Part model, mm, in its own coordinate system. Coordinates: 2 decimals unless noted, no trailing zeros. Write each loop counter-clockwise with the first axis right and the second up, starting at its lowest first coordinate (ties: lowest second). Pieces come first, ordered by that corner, then holes. Notation, with made-up numbers: M 62,-10 L 70,-10 A21 cw 70,18 Z; hole C 59,-22.5 d8. An arc over 180 degrees is marked long. Use a Markdown table: item, result. Add a question column.
Q1. Pin check, flat tip, straight feed: pin 1 Ø3 at (x, y) = (-114, -21) entering from -Z. Stop position of the tip, or through.
Q2. Slice it at A-A on x = -83. Write the cut outline in (y, z), then the cut area to 3 significant figures.
Q3. Mould opens along X. For faces 1 (the flat face through (-158, -76, 2)), 2 (the flat face through (0, -76, 2)), 3 (the cylindrical face through (-123, -105, 2)) say: released by +X, released by -X, zero draft, split by the parting line, or undercut.
Q4. Slice it at C-C on z = 1. Write the cut outline in (x, y).
Q5. Slice it at B-B on y = -97. Write the cut outline in (x, z), then the cut area to 3 significant figures.
Q6. Wall check: L1, parallel to X at y = -142.5, z = 0.9; L2, parallel to Y at x = -156, z = 2.95; L3, parallel to Y at x = -84, z = 0.7. Give the ranges that are in metal, low to high. Write a range as from..to.
from build123d import *

# Parameters (mm, degrees)
F0_W     = 158
F0_H     = 150
F1_DEPTH = 4
F2_R     = 1.5
F3_DEPTH = 25
F4_R     = 50
F5_DEPTH = 25


with BuildPart() as f1:
    # F0 (on Top) → F1 (new body)
    with BuildSketch(Plane.XY):
        with Locations((-79, -75)):
            Rectangle(F0_W, F0_H)
    extrude(amount=F1_DEPTH)

    # F2 (on face) → F3 (cut)
    with BuildSketch(Plane.XY.offset(4)):
        with Locations((-156, -142.5)):
            Circle(F2_R)
        with Locations((-2, -142.5)):
            Circle(F2_R)
        with Locations((-156, -7.5)):
            Circle(F2_R)
        with Locations((-2, -7.5)):
            Circle(F2_R)
    extrude(amount=-F3_DEPTH, mode=Mode.SUBTRACT)

    # F4 (on face) → F5 (cut)
    with BuildSketch(Plane.XY.offset(4)):
        with Locations((-83, -75)):
            Circle(F4_R)
    extrude(amount=-F5_DEPTH, mode=Mode.SUBTRACT)


solid = f1.part
Recorded:
| question | item | result |
|---|---|---|
| 1 | pin 1 | z = 0 |
| 2 | outline | M -150,0 L -125,0 L -125,4 L -150,4 Z; M -25,0 L 0,0 L 0,4 L -25,4 Z |
| 2 | area | 200 mm² |
| 3 | face 1 | released by -X |
| 3 | face 2 | released by +X |
| 3 | face 3 | undercut |
| 4 | outline | M -158,-150 L 0,-150 L 0,0 L -158,0 Z; hole C -156,-142.5 d3; hole C -156,-7.5 d3; hole C -83,-75 d100; hole C -2,-142.5 d3; hole C -2,-7.5 d3 |
| 5 | outline | M -158,0 L -127.9,0 L -127.9,4 L -158,4 Z; M -38.1,0 L 0,0 L 0,4 L -38.1,4 Z |
| 5 | area | 273 mm² |
| 6 | L1 | -158..-157.5, -154.5..-3.5, -0.5..0 |
| 6 | L2 | -150..-144, -141..-9, -6..0 |
| 6 | L3 | -150..-124.99, -25.01..0 |
